Design review of the part shown in the three views and the two pictorial views. Dimensions are in mm from the part's minimum x, y and z. A direction names the side the tool comes from. Give positions to 0.01 mm unless a question says otherwise; leave off trailing zeros. Write each loop counter-clockwise with the first axis right and the second up, starting at its lowest first coordinate (ties: lowest second). Pieces come first, ordered by that corner, then holes. Notation, with made-up numbers: M 85,41.5 L 113,41.5 A22 cw 113,74.5 Z; hole C 46.5,64.5 d7. An arc over 180 degrees is marked long. Use one line per item in the form item = value. Start each with the question number.
Q1. Mouldability with a two-part tool opening along X and no side actions: class the marked faces 4, 5, 6 and 7 as released by +X, released by -X, zero draft, split by the parting line, or undercut.
Q2. Consider section C-C on x = 35.5. Write out the cut boundary in (y, z), and give its area (3 significant figures).
Q3. For probe 1 along X at (y, z) = (14.75, 89); probe 2 along X at (y, z) = (19.75, 25.5); probe 3 along Z at (x, y) = (32.5, 5.5), list the stretches that pass through material, from the lowest coordinate up. Write a range as [from, to].
Q4. Consider section B-B on z = 58.5. Write out the cut boundary in (x, y).
Q5. Tool access review of the marked faces 1, 2 and 3: name each direction out of +Z, -Z, +X, -X, +Y, -Y from which nothing blocks a thin tool from reaching the whole face with its end or side.
Q6. Consider section A-A on y = 9. Write out the cut boundary in (x, z), and give its area (3 significant figures).
Q7. Consider section D-D on x = 95. Write out the cut boundary in (y, z).
Q8. Clearance check with flat-ended pins moving along their axes: pin 1 Ø6 at (x, y) = (88, 11) entering from -Z; pin 2 Ø12 at (x, z) = (32, 70.5) entering from -Y; pin 3 Ø16 at (y, z) = (12.5, 66.5) entering from +X. State where each tip first meets the part, or that it passes through.
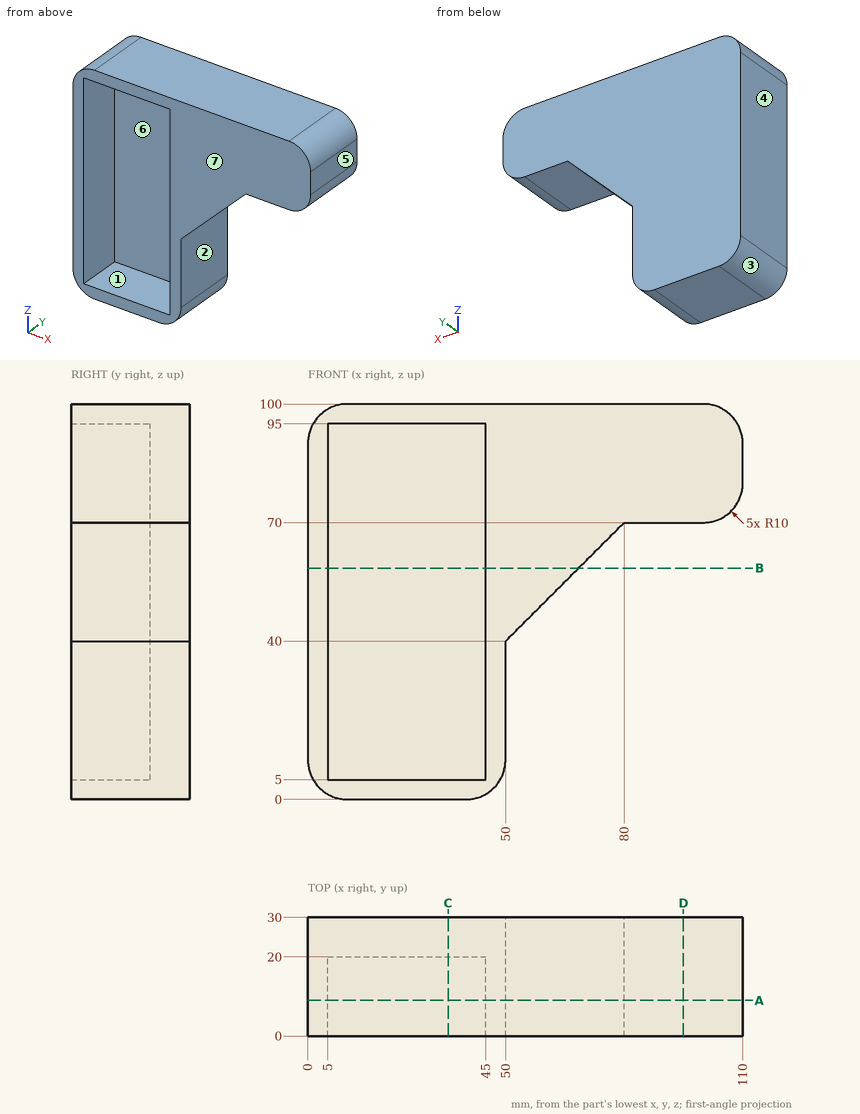
Working result:
q1.face_4 = released by -X
q1.face_5 = released by +X
q1.face_6 = undercut
q1.face_7 = zero draft
q2.outline = M 0,0 L 30,0 L 30,100 L 0,100 L 0,95 L 20,95 L 20,5 L 0,5 Z
q2.area = 1,200 mm²
q3.probe_1 = [0, 5], [45, 110]
q3.probe_2 = [0, 5], [45, 50]
q3.probe_3 = [0, 5], [95, 100]
q4.outline = M 0,0 L 5,0 L 5,20 L 45,20 L 45,0 L 68.5,0 L 68.5,30 L 0,30 Z
q5.face_1 = -Y
q5.face_2 = -Z, +X, +Y, -Y
q5.face_3 = -Z, -X, +Y, -Y
q6.outline = M 0,10 A10 ccw 10,0 L 40,0 A10 ccw 50,10 L 50,40 L 80,70 L 100,70 A10 ccw 110,80 L 110,90 A10 ccw 100,100 L 10,100 A10 ccw 0,90 Z; hole M 5,5 L 45,5 L 45,95 L 5,95 Z
q6.area = 3,540 mm²
q7.outline = M 0,70 L 30,70 L 30,100 L 0,100 Z
q8.pin_1 = 70
q8.pin_2 = 20
q8.pin_3 = 108.35
